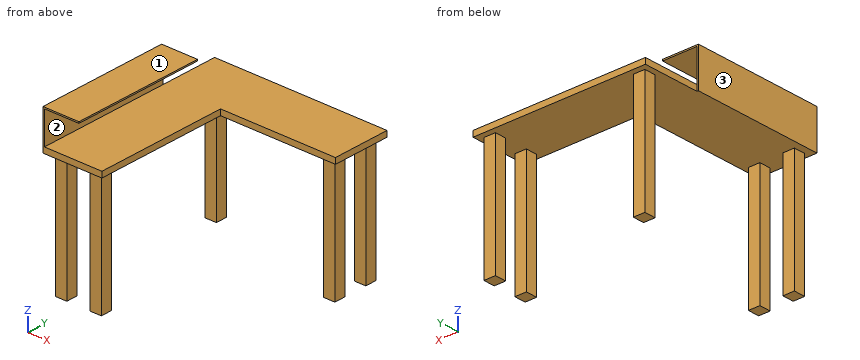
from build123d import *

# Parameters (mm, degrees)
F0_W     = 1016
F0_H     = 508
F1_DEPTH = 50.8
F2_W     = 101.6
F2_H     = 101.6
F3_DEPTH = 1066.8
F4_W     = 1168.4
F4_H     = 297.18
F4_H_2   = 50.8
F5_DEPTH = 12.7
F6_W     = 1168.4
F6_H     = 12.7
F7_DEPTH = 304.8


with BuildPart() as f1:
    # F0 (on Top) → F1 (new body)
    with BuildSketch(Plane.XY):
        Polygon((-508, 508), (-508, -1168.4), (0, -1168.4), (0, 0), (0, 508), align=None)
        with Locations((508, 254)):
            Rectangle(F0_W, F0_H)
    extrude(amount=-F1_DEPTH)

    # F2 (on face) → F3 (join)
    with BuildSketch(Plane(origin=(0, 0, -50.8), x_dir=(1, 0, 0), z_dir=(0, 0, -1))):
        with Locations((-101.6, 1066.8)):
            Rectangle(F2_W, F2_H)
        with Locations((-406.4, 1066.8)):
            Rectangle(F2_W, F2_H)
        with Locations((-406.4, -406.4)):
            Rectangle(F2_W, F2_H)
        with Locations((914.4, -101.6)):
            Rectangle(F2_W, F2_H)
        with Locations((914.4, -406.4)):
            Rectangle(F2_W, F2_H)
    extrude(amount=F3_DEPTH)

    # F4 (on face) → F5 (join)
    with BuildSketch(Plane(origin=(-508, 0, 0), x_dir=(0, -1, 0), z_dir=(-1, 0, 0))):
        with Locations((584.2, 148.59)):
            Rectangle(F4_W, F4_H)
        with Locations((584.2, -25.4)):
            Rectangle(F4_W, F4_H_2)
    extrude(amount=F5_DEPTH)

    # F6 (on face) → F7 (join)
    with BuildSketch(Plane.YZ.offset(-508)):
        with Locations((-584.2, 290.83)):
            Rectangle(F6_W, F6_H)
    extrude(amount=F7_DEPTH)


solid = f1.part
Verification items for the finished model (mm, model axes). Face numbers are marked on the shaded views. Coordinates: 2 decimals unless noted, no trailing zeros. Loops run counter-clockwise (first coordinate to the right, second up) from the corner with the lowest first, then second, coordinate; pieces in that order, holes last. Notation, with made-up numbers: M 75,11.25 L 89,11.25 A30 ccw 89,50.25 Z; hole C 31,-37.5 d10. An arc over 180 degrees is marked long. One line per item, written item: value.
1. Section check A-A on z = -476.5. Record the cut outline in (x, y), plus the area to 3 significant figures.
Answers follow:
outline: M -457.2,-1117.6 L -355.6,-1117.6 L -355.6,-1016 L -457.2,-1016 Z; M -457.2,355.6 L -355.6,355.6 L -355.6,457.2 L -457.2,457.2 Z; M -152.4,-1117.6 L -50.8,-1117.6 L -50.8,-1016 L -152.4,-1016 Z; M 863.6,50.8 L 965.2,50.8 L 965.2,152.4 L 863.6,152.4 Z; M 863.6,355.6 L 965.2,355.6 L 965.2,457.2 L 863.6,457.2 Z
area: 51,600 mm^2
2. Section check B-B on y = -665. Record the cut outline in (x, z), plus the area to 3 significant figures.
Answers follow:
outline: M -520.7,-50.8 L 0,-50.8 L 0,0 L -508,0 L -508,284.48 L -203.2,284.48 L -203.2,297.18 L -520.7,297.18 Z
area: 34,100 mm^2
3. Material ranges on line 1 along Z through (x, y) = (-265, -767); line 2 along Y through (x, z) = (867.5, -786); line 3 along Z through (x, y) = (334, 405.5), recorded low to high. Write a range as from..to.
Answers follow:
line 1: -50.8..0, 284.48..297.18
line 2: 50.8..152.4, 355.6..457.2
line 3: -50.8..0
4. Mould release check, pull along Z, two halves, no side actions. Record for the marked faces 1, 2 and 3: pulls with the +Z half, pulls with the -Z half, needs draft (parallel to the pull), parting line crosses it, or undercut.
Answers follow:
face 1: pulls with the +Z half
face 2: undercut
face 3: needs draft
5. Section check C-C on x = 705.5. Record the cut outline in (y, z), plus the area to 3 significant figures.
Answers follow:
outline: M 0,-50.8 L 508,-50.8 L 508,0 L 0,0 Z
area: 25,800 mm^2
6. Gauge pin test, flat ends, axial feed: P1, Ø1.5, axis at x = 417, y = 78.5, coming from the +Z side; P2, Ø6.5, axis at y = -409, z = 290, coming from the +X side. Record the tip position at first contact, or that the pin passes through.
Answers follow:
P1: z = 0
P2: x = -203.2
7. Section check D-D on y = 397.5. Record the cut outline in (x, z).
Answers follow:
outline: M -508,-50.8 L -457.2,-50.8 L -457.2,-1117.6 L -355.6,-1117.6 L -355.6,-50.8 L 863.6,-50.8 L 863.6,-1117.6 L 965.2,-1117.6 L 965.2,-50.8 L 1016,-50.8 L 1016,0 L -508,0 Z
